Design review of the part built by this model. Coordinates are the model's own, in mm. A direction names the side the tool comes from. Give positions to 0.01 mm unless a question says otherwise; leave off trailing zeros. Write each loop counter-clockwise with the first axis right and the second up, starting at its lowest first coordinate (ties: lowest second). Pieces come first, ordered by that corner, then holes. Notation, with made-up numbers: (31, 68) -> (63, 68) arc R17 ccw to (63, 88) -> close; hole circle Ø9 at (71.5, 72.25). An arc over 180 degrees is marked (long way). Answer as a JSON object with one key per item and string values.
```python
from build123d import *

# Parameters (mm, degrees)
F1_DEPTH = 5.2
F2_T     = -0.5


with BuildPart() as f1:
    # F0 (on Top) → F1 (new body)
    with BuildSketch(Plane.XY):
        with BuildLine():
            ThreePointArc((36.2717987143, 8.2581243652), (35.9383049337, 8.8032091706), (35.3428416161, 9.0350690081))
            ThreePointArc((35.3428416161, 9.0350690081), (0, 9.85), (-35.3428416161, 9.0350690081))
            ThreePointArc((-35.3428416161, 9.0350690081), (-35.9383049337, 8.8032091706), (-36.2717987143, 8.2581243652))
            ThreePointArc((-36.2717987143, 8.2581243652), (-37.2, 0), (-36.2717987143, -8.2581243652))
            ThreePointArc((-36.2717987143, -8.2581243652), (-35.9383049337, -8.8032091706), (-35.3428416161, -9.0350690081))
            ThreePointArc((-35.3428416161, -9.0350690081), (0, -9.85), (35.3428416161, -9.0350690081))
            ThreePointArc((35.3428416161, -9.0350690081), (35.9383049337, -8.8032091706), (36.2717987143, -8.2581243652))
            ThreePointArc((36.2717987143, -8.2581243652), (37.2, 0), (36.2717987143, 8.2581243652))
        make_face()
    extrude(amount=F1_DEPTH)

    # F2
    f2_openings = [f1.faces().sort_by_distance(p)[0] for p in [
        (0, 0, 0),
    ]]
    offset(amount=F2_T, openings=f2_openings)

    # F5 (on Front) → F6 (revolve)
    with BuildSketch(Plane.XZ):
        with BuildLine():
            Line((15.87, 5.2), (18.37, 5.2))
            ThreePointArc((18.37, 5.2), (17.637766953, 6.967766953), (15.87, 7.7))
            Line((15.87, 7.7), (15.87, 5.2))
        make_face()
    revolve(axis=Axis((15.87, 0, 7.7), (0, 0, 1)))

    # F5 (on Front) → F7 (revolve)
    with BuildSketch(Plane.XZ):
        with BuildLine():
            Line((-26.45, 5.2), (-23.95, 5.2))
            ThreePointArc((-23.95, 5.2), (-24.682233047, 6.967766953), (-26.45, 7.7))
            Line((-26.45, 7.7), (-26.45, 5.2))
        make_face()
    revolve(axis=Axis((-26.45, 0, 7.7), (0, 0, 1)))

    # F5 (on Front) → F8 (revolve)
    with BuildSketch(Plane.XZ):
        with BuildLine():
            Line((-15.87, 5.2), (-13.37, 5.2))
            ThreePointArc((-13.37, 5.2), (-14.102233047, 6.967766953), (-15.87, 7.7))
            Line((-15.87, 7.7), (-15.87, 5.2))
        make_face()
    revolve(axis=Axis((-15.87, 0, 7.7), (0, 0, 1)))

    # F5 (on Front) → F9 (revolve)
    with BuildSketch(Plane.XZ):
        with BuildLine():
            Line((-5.29, 5.2), (-2.79, 5.2))
            ThreePointArc((-2.79, 5.2), (-3.522233047, 6.967766953), (-5.29, 7.7))
            Line((-5.29, 7.7), (-5.29, 5.2))
        make_face()
    revolve(axis=Axis((-5.29, 0, 7.7), (0, 0, 1)))

    # F5 (on Front) → F10 (revolve)
    with BuildSketch(Plane.XZ):
        with BuildLine():
            Line((5.29, 5.2), (7.79, 5.2))
            ThreePointArc((7.79, 5.2), (7.057766953, 6.967766953), (5.29, 7.7))
            Line((5.29, 7.7), (5.29, 5.2))
        make_face()
    revolve(axis=Axis((5.29, 0, 7.7), (0, 0, 1)))

    # F5 (on Front) → F11 (revolve)
    with BuildSketch(Plane.XZ):
        with BuildLine():
            Line((26.45, 5.2), (28.95, 5.2))
            ThreePointArc((28.95, 5.2), (28.217766953, 6.967766953), (26.45, 7.7))
            Line((26.45, 7.7), (26.45, 5.2))
        make_face()
    revolve(axis=Axis((26.45, 0, 7.7), (0, 0, 1)))


solid = f1.part
```
(1) Clearance check with flat-ended pins moving along their axes: pin 1 (9.5 mm diameter, centred on x = -7.5, y = 4, fed in from -Z); pin 2 (1 mm diameter, centred on y = 3, z = 2, fed in from +X); pin 3 (1 mm diameter, centred on x = 13.5, z = 5.5, fed in from +Y). State where each tip first meets the part, or that it passes through.
Here are the results:
{"pin 1": "stops at z = 4.7", "pin 2": "stops at x = 37.12", "pin 3": "stops at y = 9.74"}
(2) The part is to be moulded in two halves that separate along X. For faces 4 (the cylindrical face through (0.49, 9.35, 2.32)), 5 (the cylindrical face through (-37.2, 0.1, 2.6)), 6 (the cylindrical face through (37.2, -0.1, 2.6)), 7 (the cylindrical face through (-36.7, 0.1, 2.3)), say which applies: +X half, -X half, draft (parallel to the pull), parting line (faces both ways), or undercut.
Here are the results:
{"face 4": "undercut", "face 5": "-X half", "face 6": "+X half", "face 7": "undercut"}
(3) We need section B-B, the plane x = 22. State the section outline as (y, z) points.
Here are the results:
{"outline": "(-9.53, 0) -> (-9.03, 0) -> (-9.03, 4.7) -> (9.03, 4.7) -> (9.03, 0) -> (9.53, 0) -> (9.53, 5.2) -> (-9.53, 5.2) -> close"}
(4) We need section D-D, the plane y = 6. State the section outline as (x, z) points, then the cut area to 3 significant figures.
Here are the results:
{"outline": "(-36.71, 0) -> (-36.21, 0) -> (-36.21, 4.7) -> (36.21, 4.7) -> (36.21, 0) -> (36.71, 0) -> (36.71, 5.2) -> (-36.71, 5.2) -> close", "area": "41.5 mm²"}
(5) We need section A-A, the plane z = 3. State the section outline as (x, y) points, then the cut area to 3 significant figures.
Here are the results:
{"outline": "(-36.27, -8.26) arc R1 ccw to (-35.34, -9.04) arc R766.8 ccw to (35.34, -9.04) arc R1 ccw to (36.27, -8.26) arc R37.2 ccw to (36.27, 8.26) arc R1 ccw to (35.34, 9.04) arc R766.8 ccw to (-35.34, 9.04) arc R1 ccw to (-36.27, 8.26) arc R37.2 ccw to start; hole (-35.78, -8.15) arc R0.5 ccw to (-35.32, -8.54) arc R766.3 ccw to (35.32, -8.54) arc R0.5 ccw to (35.78, -8.15) arc R36.7 ccw to (35.78, 8.15) arc R0.5 ccw to (35.32, 8.54) arc R766.3 ccw to (-35.32, 8.54) arc R0.5 ccw to (-35.78, 8.15) arc R36.7 ccw to start", "area": "89.2 mm²"}
(6) For line 1 along Y through (x, z) = (3, 4); line 2 along X through (y, z) = (0.5, 1.75); line 3 along Z through (x, y) = (-25.5, -8), list the stretches that pass through material, from the lowest coordinate up.
Here are the results:
{"line 1": "y = -9.84 to -9.34, 9.34 to 9.84", "line 2": "x = -37.2 to -36.7, 36.7 to 37.2", "line 3": "z = 4.7 to 5.2"}
(7) For faces 1 (the cylindrical face through (0.49, 9.85, 2.56)), 2 (the flat face through (-1, 0, 5.2)), 3 (the cylindrical face through (-0.49, -9.35, 2.32)), list the 3-axis set-ups (+Z, -Z, +X, -X, +Y, -Y) from which the entire face can be reached by the end or side of a thin tool; tool diameter is ignored.
Here are the results:
{"face 1": "+Z, -Z, +Y", "face 2": "+Z", "face 3": "-Z"}
(8) We need section C-C, the plane z = 6.5. State the section outline as (x, y) points, then the cut area to 3 significant figures.
Here are the results:
{"outline": "circle Ø4.27 at (-26.45, 0); circle Ø4.27 at (-15.87, 0); circle Ø4.27 at (-5.29, 0); circle Ø4.27 at (5.29, 0); circle Ø4.27 at (15.87, 0); circle Ø4.27 at (26.45, 0)", "area": "86.0 mm²"}
